Input: part model. Units: mm. Frame: model coordinates. Face numbers are marked on the shaded views. A direction names the side the tool comes from. Round coordinates to 2 decimals unless told otherwise and drop trailing zeros. Loops run counter-clockwise (first coordinate to the right, second up) from the corner with the lowest first, then second, coordinate; pieces in that order, holes last. Notation, with made-up numbers: (29.25, -6) -> (47.25, -6) arc R33 cw to (47.25, 22) -> close; hole circle Ø6 at (54.25, 29). An arc over 180 degrees is marked (long way). Answer in a Markdown table with one row per item. Add a question column.
Q1. Section B-B, the plane z = 7.75. Output: boundary loops of the cut face in (x, y).
Q2. Pin query (flat end, axial travel): pin 1 (4 mm diameter, centred on x = 0, y = -6.46, fed in from +Z); pin 2 (2 mm diameter, centred on y = -8, z = 13.5, fed in from -X); pin 3 (1.1 mm diameter, centred on y = -6.46, z = 3, fed in from -X); pin 4 (3 mm diameter, centred on x = -2, z = 5.5, fed in from +Y). Return the tip coordinate at first contact, or that it passes through.
Q3. Reachability of the marked faces 1 and 2 from +Z, -Z, +X, -X, +Y, -Y: full face, straight path, thin tool, end or side. Return the list, or none.
Q4. Section A-A, the plane z = 23. Output: boundary loops of the cut face in (x, y).
Q5. Ray query, L1, parallel to Y at x = 0, z = 23.75; L2, parallel to Y at x = 0, z = 3.5; L3, parallel to Z at x = -1.25, y = -5.75. Return the intervals inside material, ascending. Write a range as from..to.
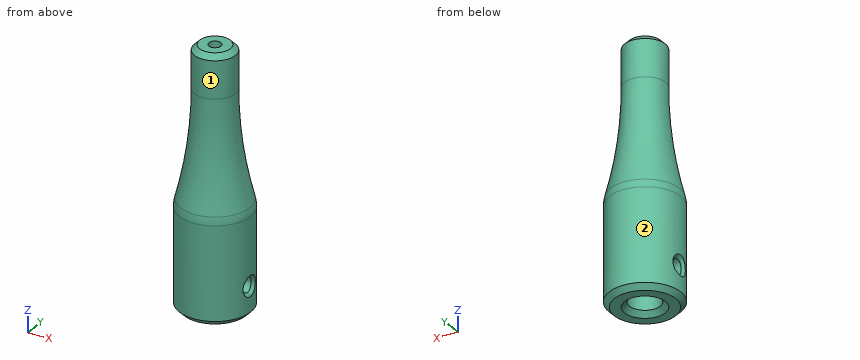
Autodesk Inventor part; units mm, degrees
ref_plane "YZ Plane" through (0, 0, 0) normal (1, 0, 0) x (0, 1, 0)
ref_plane "XZ Plane" through (0, 0, 0) normal (0, 1, 0) x (-1, 0, 0)
ref_plane "XY Plane" through (0, 0, 0) normal (0, 0, 1) x (1, 0, 0)
sketch "Sketch1" plane through (0, 0, 0) normal (0, 0, 1) x (1, 0, 0)
  circle A0 centre (0, -6.4566) radius 1.5
  circle A1 centre (0, -6.4566) radius 1.5
  circle A2 centre (0, -6.4566) radius 3.5
  point P0 (0, 0)
  dimension "d0" = 3
  dimension "d1" = 7
extrude "Extrusion1" add sketch "Sketch1" along normal blind 8
sketch "Sketch2" plane through (0, -6.4566, 8) normal (0, 0, 1) x (1, 0, 0)
  circle A0 centre (0, 0) radius 3.5
  point P0 (0, 6.4566)
extrude "Extrusion2" add sketch "Sketch2" along normal blind 2
sketch "Sketch3" plane through (0, -6.4566, 10) normal (0, 0, 1) x (1, 0, 0)
  circle A0 centre (0, 0) radius 3.5
  circle A1 centre (0, 0) radius 0.6
  circle A2 centre (0, 0) radius 2
  point P0 (0, 6.4566)
  dimension "d6" = 1.2
  dimension "d7" = 4
extrude "Extrusion3" add sketch "Sketch3" along normal blind 15 contours A2
fillet "Fillet1" radius 40 1 edges at (-2, -6.4566, 10)
fillet "Fillet2" radius 3 1 edges at (-3.5, -6.4566, 10)
chamfer "Chamfer1" distance 0.5 angle 45 1 edges at (-1.5, -6.4566, 0)
chamfer "Chamfer2" distance 0.5 angle 45 1 edges at (-2, -6.4566, 25)
sketch "Sketch4" plane through (0, 0, 0) normal (1, 0, 0) x (0, 1, 0)
  line L0 (-2.9566, 0) -> (-9.9566, 0)
  line L1 (-6.4566, 0) -> (-6.4566, 3)
  circle A0 centre (-6.4566, 3) radius 0.7
  point P0 (0, 0)
  dimension "d18" = 3
  dimension "d19" = 1.4
extrude "Extrusion4" cut sketch "Sketch4" along normal mid plane 15
chamfer "Chamfer3" distance 0.3 angle 45 4 edges at (3.4625, -5.9454, 3.4781) (3.4627, -5.9468, 2.5204) (3.4293, -7.1566, 2.9993) (-3.4293, -7.1565, 2.9852)
chamfer "Chamfer4" distance 0.5 angle 45 1 edges at (-3.5, -6.4566, 0)
properties part number "needle_conn_1"
Answer block:
| question | item | result |
|---|---|---|
| 1 | outline | circle Ø7 at (0, -6.46); hole circle Ø3 at (0, -6.46) |
| 2 | pin 1 | z = 25 |
| 2 | pin 2 | x = -2.7 |
| 2 | pin 3 | through |
| 2 | pin 4 | y = -2.99 |
| 3 | face 1 | +Z |
| 3 | face 2 | +Z, -Z |
| 4 | outline | circle Ø4 at (0, -6.46); hole circle Ø1.2 at (0, -6.46) |
| 5 | L1 | -8.46..-7.06, -5.86..-4.46 |
| 5 | L2 | -9.96..-7.96, -4.96..-2.96 |
| 5 | L3 | 8..25 |
